Can you work these out from the model? Positions are in its coordinate system, mm. A direction names the side the tool comes from. Round coordinates to 2 decimals unless told otherwise and drop trailing zeros. Order: outer loops, then holes, each group sorted by start corner. A loop starts at its lowest first (then second) coordinate and runs counter-clockwise, first axis right, second up.
Q1. If we section it at D-D (x = 48.5): Please give me the cut outline in (y, z), plus the area to 3 significant figures.
Q2. If we section it at C-C (y = 5): Please give me the cut outline in (x, z).
Q3. If we section it at A-A (y = 23.5): Please give me the cut outline in (x, z), plus the area to 3 significant figures.
Q4. We'd pull the mould along Z, two halves only. Please class faces 4 (the face through (-86, 18, 0)), 5 (the face through (-1, 2, 0)), 6 (the face through (-1, 10, -28.5)): pulls with the +Z half, pulls with the -Z half, needs draft (parallel to the pull), parting line crosses it, or undercut.
Q5. For faces 1 (the face through (86, 18, 0)), 2 (the face through (72, 28, 28)), 3 (the face through (-84, 19, 0)), which set-ups out of +Z, -Z, +X, -X, +Y, -Y let a thin tool reach every point of the face, with its end or its side?
Q6. Will these pins go through, and if not, where does the flat tip stop? P1, Ø5, axis at x = -9.5, z = -12.5, coming from the +Y side; P2, Ø1, axis at x = 9.5, z = 28, coming from the +Y side.
Q7. If we section it at B-B (z = 16.5): Please give me the cut outline in (x, y).
Q8. If I drill on line 1 (X direction, y = 19, z = 2); line 2 (Z direction, x = -77, y = 12); line 3 (Y direction, x = 76.5, z = -1), over which ranges is the centre line in solid material (lowest first)?
from build123d import *

# Parameters (mm, degrees)
SKETCH_1_W          = 172
SKETCH_1_H          = 57
EXTRUDE_1_DEPTH     = 2
SKETCH_3_W          = 172
SKETCH_3_H          = 57
SKETCH_3_W_2        = 168
SKETCH_3_H_2        = 53
EXTRUDE_2_DEPTH     = 35
CUT_EXTRUDE_1_DEPTH = 110.608393839


with BuildPart() as part:
    # 草图1 → 凸台-拉伸1 (new body)
    with BuildSketch(Plane(origin=(0, 0, 0), x_dir=(1, 0, 0), z_dir=(0, 1, 0))):
        Rectangle(SKETCH_1_W, SKETCH_1_H)
    extrude(amount=EXTRUDE_1_DEPTH)

    # 草图3 → 凸台-拉伸2 (add)
    with BuildSketch(Plane(origin=(0, 2, 0), x_dir=(1, 0, 0), z_dir=(0, 1, 0))):
        Rectangle(SKETCH_3_W, SKETCH_3_H)
        Rectangle(SKETCH_3_W_2, SKETCH_3_H_2, mode=Mode.SUBTRACT)
    extrude(amount=EXTRUDE_2_DEPTH)

    # 草图4 → 切除-拉伸1 (cut, through all)
    with BuildSketch(Plane.XY.offset(28.5)):
        Polygon((-81, 37), (-64, 20), (64, 20), (81, 37), align=None)
    extrude(amount=-CUT_EXTRUDE_1_DEPTH, mode=Mode.SUBTRACT)


solid = part.part
Solution:
1. outline: (0, -28.5) - (20, -28.5) - (20, -26.5) - (2, -26.5) - (2, 26.5) - (20, 26.5) - (20, 28.5) - (0, 28.5) - close
1. area: 186 mm2
2. outline: (-86, -28.5) - (86, -28.5) - (86, 28.5) - (-86, 28.5) - close; hole (-84, -26.5) - (84, -26.5) - (84, 26.5) - (-84, 26.5) - close
3. outline: (-86, -28.5) - (-67.5, -28.5) - (-67.5, -26.5) - (-84, -26.5) - (-84, 26.5) - (-67.5, 26.5) - (-67.5, 28.5) - (-86, 28.5) - close; (67.5, -28.5) - (86, -28.5) - (86, 28.5) - (67.5, 28.5) - (67.5, 26.5) - (84, 26.5) - (84, -26.5) - (67.5, -26.5) - close
3. area: 360 mm2
4. face 4: needs draft
4. face 5: undercut
4. face 6: pulls with the -Z half
5. face 1: +Z, -Z, +X, +Y, -Y
5. face 2: +Z, -Z, +Y
5. face 3: +Y
6. P1: stops at y = 2
6. P2: stops at y = 20
7. outline: (-86, 0) - (86, 0) - (86, 37) - (84, 37) - (84, 2) - (-84, 2) - (-84, 37) - (-86, 37) - close
8. line 1: x = -86 to -84, 84 to 86
8. line 2: z = -28.5 to -26.5, 26.5 to 28.5
8. line 3: y = 0 to 2
